from build123d import *

# Parameters (mm, degrees)
EXTRUDE_2_DEPTH     = 20
EXTRUDE_1_DEPTH     = 3
EXTRUDE_2_2_DEPTH   = 3
CUT_EXTRUDE_1_DEPTH = 34
CUT_EXTRUDE_2_DEPTH = 34


with BuildPart() as part:
    # 草图1 → Extrude 2 (new body)
    with BuildSketch(Plane(origin=(0, 0, 0), x_dir=(1, 0, 0), z_dir=(0, 1, 0))):
        Polygon((0, 20), (0, 0), (20, 0), (20, 3), (3, 3), (3, 20), align=None)
    extrude(amount=EXTRUDE_2_DEPTH)

    # 草图2 → 凸台-拉伸1 (add)
    with BuildSketch(Plane(origin=(0, 20, 0), x_dir=(1, 0, 0), z_dir=(0, 1, 0))):
        Polygon((3, 20), (20, 3), (20, 0), (0, 0), (0, 20), align=None)
    extrude(amount=-EXTRUDE_1_DEPTH)

    # 草图3 → Extrude 2 2 (add)
    with BuildSketch(Plane.XZ):
        Polygon((20, -3), (3, -20), (3, -3), align=None)
    extrude(amount=-EXTRUDE_2_2_DEPTH)

    # 草图5 → 切除-拉伸1 (cut, through all)
    with BuildSketch(Plane(origin=(0, 0, -3), x_dir=(-1, 0, 0), z_dir=(0, 0, -1))):
        with BuildLine():
            Line((-7.5, 8), (-12.5, 8))
            ThreePointArc((-12.5, 8), (-14.5, 10), (-12.5, 12))
            Line((-12.5, 12), (-7.5, 12))
            ThreePointArc((-7.5, 12), (-5.5, 10), (-7.5, 8))
        make_face()
    extrude(amount=-CUT_EXTRUDE_1_DEPTH, mode=Mode.SUBTRACT)

    # 草图6 → 切除-拉伸2 (cut, through all)
    with BuildSketch(Plane(origin=(3, 0, 0), x_dir=(0, 0, -1), z_dir=(1, 0, 0))):
        with BuildLine():
            Line((7.5, 12), (12.5, 12))
            ThreePointArc((12.5, 12), (14.5, 10), (12.5, 8))
            Line((12.5, 8), (7.5, 8))
            ThreePointArc((7.5, 8), (5.5, 10), (7.5, 12))
        make_face()
    extrude(amount=-CUT_EXTRUDE_2_DEPTH, mode=Mode.SUBTRACT)


solid = part.part
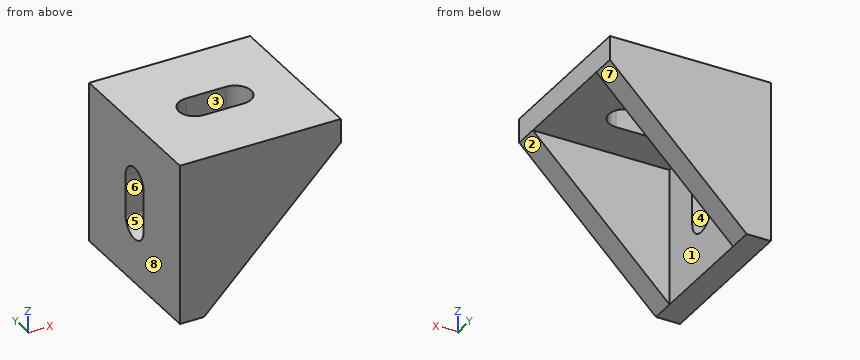
Part model, mm, in its own coordinate system. Face numbers are marked on the shaded views. A direction names the side the tool comes from. Give positions to 0.01 mm unless a question says otherwise; leave off trailing zeros. Order: outer loops, then holes, each group sorted by start corner. A loop starts at its lowest first (then second) coordinate and runs counter-clockwise, first axis right, second up. Notation, with made-up numbers: (71.5, 54) - (108.5, 54) arc R35 ccw to (108.5, 88) - close; hole circle Ø10 at (82.5, 57). An arc over 180 degrees is marked (long way). One line per question, with ' | ' between items.
1. Band-saw the part on C-C on z = -2.25. List the corners of the cut face in (x, y), then the cut area to 3 significant figures.
Filled in:
outline: (0, 0) - (20, 0) - (20, 20) - (0, 20) - close; hole (7.5, 8) - (12.5, 8) arc R2 ccw to (12.5, 12) - (7.5, 12) arc R2 ccw to start | area: 367 mm²
2. Band-saw the part on B-B on z = -10.5. List the corners of the cut face in (x, y).
Filled in:
outline: (0, 0) - (12.5, 0) - (12.5, 3) - (3, 3) - (3, 8) - (0, 8) - close; (0, 12) - (3, 12) - (3, 17) - (12.5, 17) - (12.5, 20) - (0, 20) - close
3. Band-saw the part on A-A on y = 10. List the corners of the cut face in (x, z).
Filled in:
outline: (0, -20) - (3, -20) - (3, -14.5) - (0, -14.5) - close; (0, -5.5) - (3, -5.5) - (3, -3) - (5.5, -3) - (5.5, 0) - (0, 0) - close; (14.5, -3) - (20, -3) - (20, 0) - (14.5, 0) - close
4. Pull direction Z, two halves, no side cores. Call the marked faces 5, 6, 7 and 8: +Z half, -Z half, draft (parallel to the pull), parting line (faces both ways), or undercut.
Filled in:
face 5: undercut | face 6: undercut | face 7: -Z half | face 8: draft
5. Which spindle directions (+Z, -Z, +X, -X, +Y, -Y) get a long thin tool onto all of the face, cutting with end or side? Do the marked faces 1, 2, 3 and 4. Say none if no direction does.
Filled in:
face 1: -Z, +X | face 2: -Z, +X, +Y, -Y | face 3: +Z, -Z | face 4: +X, -X
6. Drill centre lines: probe 1 along Y at (x, z) = (5, -15); probe 2 along X at (y, z) = (12.5, -17.25); probe 3 along Y at (x, z) = (9.75, -1). Where is each one in solid material? Low to high.
Filled in:
probe 1: 0 to 3, 17 to 20 | probe 2: 0 to 3 | probe 3: 0 to 8, 12 to 20
7. Band-saw the part on D-D on x = 10.5. List the corners of the cut face in (y, z).
Filled in:
outline: (0, -12.5) - (3, -12.5) - (3, -3) - (8, -3) - (8, 0) - (0, 0) - close; (12, -3) - (17, -3) - (17, -12.5) - (20, -12.5) - (20, 0) - (12, 0) - close
8. Drop a flat-ended pin along its axis: P1, Ø4, axis at y = 9, z = -10, coming from the +X side. Give the stop position or say it passes through.
Filled in:
P1: x = 3
